For this review, use the dimensioned drawing (mm, ordinates from the lowest corner) and the shaded views. A direction names the side the tool comes from. Coordinates: 2 decimals unless noted, no trailing zeros. Loops run counter-clockwise (first coordinate to the right, second up) from the corner with the lowest first, then second, coordinate; pieces in that order, holes last. Notation, with made-up numbers: M 44.5,23 L 48.5,23 A24 ccw 48.5,54 Z; hole C -37.75,15 d4. An arc over 180 degrees is marked long. One line per item, written item: value.
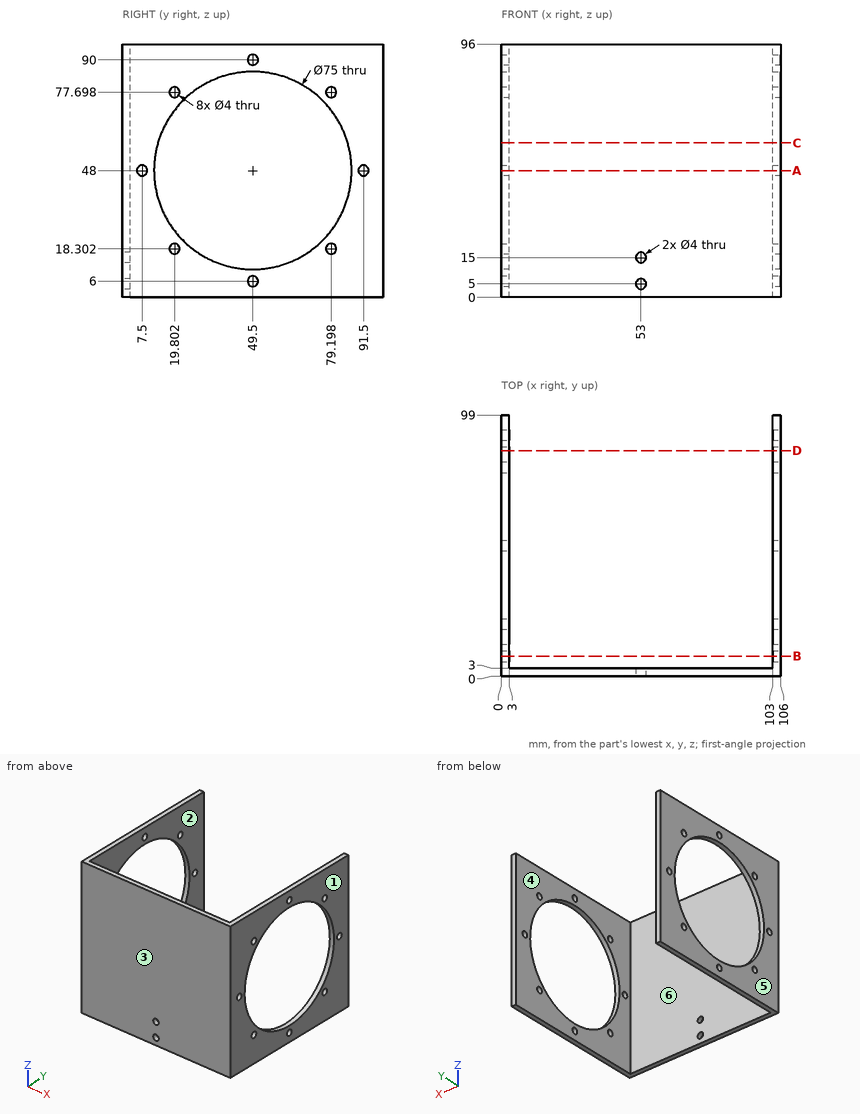
(1) Add section B-B on y = 7.5. State the section outline as (x, z) points, then the cut area to 3 significant figures.
Checks:
outline: M 0,0 L 3,0 L 3,46 L 0,46 Z; M 0,50 L 3,50 L 3,96 L 0,96 Z; M 103,0 L 106,0 L 106,46 L 103,46 Z; M 103,50 L 106,50 L 106,96 L 103,96 Z
area: 552 mm^2
(2) Add section C-C on z = 58.5. State the section outline as (x, y) points, then the cut area to 3 significant figures.
Checks:
outline: M 0,0 L 106,0 L 106,13.5 L 103,13.5 L 103,3 L 3,3 L 3,13.5 L 0,13.5 Z; M 0,85.5 L 3,85.5 L 3,99 L 0,99 Z; M 103,85.5 L 106,85.5 L 106,99 L 103,99 Z
area: 462 mm^2
(3) Draft analysis for pull direction X (two halves, no side actions). For the marked faces 1, 2, 3 and 4, state which applies: pulls with the +X half, pulls with the -X half, needs draft (parallel to the pull), parting line crosses it, or undercut.
Checks:
face 1: pulls with the +X half
face 2: undercut
face 3: needs draft
face 4: undercut
(4) Tool access review of the marked faces 5 and 6: name each direction out of +Z, -Z, +X, -X, +Y, -Y from which nothing blocks a thin tool from reaching the whole face with its end or side.
Checks:
face 5: +Z, -Z, -X, +Y, -Y
face 6: +Z, -Z, +Y
(5) To check wall thickness, follow L1, parallel to X at y = 90.5, z = 33; L2, parallel to Y at x = 104.05, z = 90; L3, parallel to Y at x = 12, z = 34. State the ranges of each line that lie inside material, in increasing order. Write a range as [from, to].
Checks:
L1: [0, 3], [103, 106]
L2: [0, 47.5], [51.5, 99]
L3: [0, 3]
(6) Add section A-A on z = 48. State how many separate pieces and enclosed holes the cut face has, then the cut area to 3 significant figures.
Checks:
separate pieces: 7
enclosed holes: 0
area: 396 mm^2
(7) Add section D-D on y = 85.5. State the section outline as (x, z) points, then the cut area to 3 significant figures.
Checks:
outline: M 0,0 L 3,0 L 3,37.5 L 0,37.5 Z; M 0,58.5 L 3,58.5 L 3,96 L 0,96 Z; M 103,0 L 106,0 L 106,37.5 L 103,37.5 Z; M 103,58.5 L 106,58.5 L 106,96 L 103,96 Z
area: 450 mm^2
(8) Insertion check: pin 1 Ø3.5 at (y, z) = (7.5, 48) entering from -X; pin 2 Ø6 at (x, z) = (53.5, 83.5) entering from +Y. Each pin has a flat end and moves straight along its axis. Give the tip position at first contact, or say it passes through.
Checks:
pin 1: through
pin 2: y = 3
